from build123d import *

# Parameters (mm, degrees)
BODY_SKETCH_W                                = 46
BODY_SKETCH_H                                = 17
BODY_DEPTH                                   = 105
BODY_ROD_HOLES_SKETCH_R                      = 3
BODY_ROD_HOLES_DEPTH                         = 10
BODY_PISTON_HOLES_SKETCH_R                   = 4.05
BODY_PISTON_HOLES_DEPTH                      = 51
TOP_SWITCH_GROOVES_DEPTH                     = 108.953693777
SHCS_MGT_HOLE_CHAM_SIZE                      = 0.3
SHCS_MGT_HOLE_PAT_COUNT                      = 2
SHCS_MGT_HOLE_PAT_PITCH                      = 40
SHCS_MGT_HOLE_CHAM_OF_SHCS_MGT_HOLE_PAT_SIZE = 0.3
SHCS_MGT_HOLE_BOT_TAP_AT_2_COUNT             = 2
SHCS_MGT_HOLE_BOT_TAP_AT_2_PITCH             = 40
ADJUSTER_NUT_DEPTH                           = 9
ADJUSTER_NUT_THREADS_SKETCH_W                = 1.4
ADJUSTER_NUT_THREADS_SKETCH_H                = 17
TAP_DRILL_FOR_M5X0_8_TAP1_D                  = 4.2
TAP_DRILL_FOR_M5X0_8_TAP1_DEPTH              = 4.5
TAP_DRILL_FOR_M5X0_8_TAP1_CSINK_D            = 5
TAP_DRILL_FOR_M5X0_8_TAP1_CSINK_ANGLE        = 90
TAP_DRILL_FOR_M5X0_8_TAP1_TIP                = 1.2618073
TAP_DRILL_FOR_M5X0_8_TAP2_D                  = 4.2
TAP_DRILL_FOR_M5X0_8_TAP2_DEPTH              = 4.5
TAP_DRILL_FOR_M5X0_8_TAP2_CSINK_D            = 5
TAP_DRILL_FOR_M5X0_8_TAP2_CSINK_ANGLE        = 90
TAP_DRILL_FOR_M5X0_8_TAP2_TIP                = 1.2618073
MOUNT_HOLES_1_D                              = 2.5
MOUNT_HOLES_1_DEPTH                          = 4.5
MOUNT_HOLES_1_CSINK_D                        = 3
MOUNT_HOLES_1_CSINK_ANGLE                    = 90
MOUNT_HOLES_1_TIP                            = 0.751075774
MOUNT_HOLES_2_D                              = 2.5
MOUNT_HOLES_2_DEPTH                          = 4.5
MOUNT_HOLES_2_CSINK_D                        = 3
MOUNT_HOLES_2_CSINK_ANGLE                    = 90
MOUNT_HOLES_2_TIP                            = 0.751075774


with BuildPart() as part:
    # Body_Sketch → Body (new body)
    with BuildSketch(Plane(origin=(0, 0, 0), x_dir=(0, 0, -1), z_dir=(1, 0, 0))):
        with Locations((0, 1.5)):
            Rectangle(BODY_SKETCH_W, BODY_SKETCH_H)
    extrude(amount=BODY_DEPTH)

    # Body Rod Holes_Sketch → Body Rod Holes (cut)
    with BuildSketch(Plane.ZY):
        with Locations((-10, 0)):
            Circle(BODY_ROD_HOLES_SKETCH_R)
        with Locations(Location((10, 0, 0), (0, 0, 180))):
            Circle(BODY_ROD_HOLES_SKETCH_R)
    extrude(amount=-BODY_ROD_HOLES_DEPTH, mode=Mode.SUBTRACT)

    # Body Piston Holes_Sketch → Body Piston Holes (cut)
    with BuildSketch(Plane.ZY.offset(-10)):
        with Locations((10, 0)):
            Circle(BODY_PISTON_HOLES_SKETCH_R)
        with Locations((-10, 0)):
            Circle(BODY_PISTON_HOLES_SKETCH_R)
    extrude(amount=-BODY_PISTON_HOLES_DEPTH, mode=Mode.SUBTRACT)

    # Top Switch Grooves_Sketch → Top Switch Grooves (cut, through all)
    with BuildSketch(Plane.ZY):
        Polygon((13.65, 5.2), (19.95, 5.2), (19.95, 8.8), (19.3, 9.175277675), (19.3, 10), (14.3, 10), (14.3, 9.175277675), (13.65, 8.8), align=None)
        Polygon((-13.65, 8.8), (-13.65, 5.2), (-19.95, 5.2), (-19.95, 8.8), (-19.3, 9.175277675), (-19.3, 10), (-14.3, 10), (-14.3, 9.175277675), align=None)
    extrude(amount=-TOP_SWITCH_GROOVES_DEPTH, mode=Mode.SUBTRACT)

    # SHCS MGT Hole_Sketch → SHCS MGT Hole (revolve, cut)
    with BuildSketch(Plane.XY, mode=Mode.PRIVATE) as shcs_mgt_hole_sk:
        Polygon((20, 10), (16.75, 10), (16.75, 6.7), (18.3, 6.7), (18.3, -7), (20, -7), align=None)
    shcs_mgt_hole = revolve(shcs_mgt_hole_sk.sketch.rotate(Axis((20, -11.506886035, 0), (0, 1, 0)), 270), axis=Axis((20, -11.506886035, 0), (0, 1, 0)), mode=Mode.SUBTRACT)

    # SHCS MGT Hole Cham
    shcs_mgt_hole_cham_edges = [part.edges().sort_by_distance(p)[0] for p in [
        (20, 10, 3.25),
    ]]
    chamfer(shcs_mgt_hole_cham_edges, length=SHCS_MGT_HOLE_CHAM_SIZE)

    # SHCS MGT Hole Pat: SHCS MGT Hole ×2
    with Locations(*[(i * SHCS_MGT_HOLE_PAT_PITCH, 0, 0) for i in range(1, SHCS_MGT_HOLE_PAT_COUNT)]):
        add(shcs_mgt_hole, mode=Mode.SUBTRACT)

    # SHCS MGT Hole Cham of SHCS MGT Hole Pat
    shcs_mgt_hole_cham_of_shcs_mgt_hole_pat_edges = [part.edges().sort_by_distance(p)[0] for p in [
        (60, 10, 3.25),
    ]]
    chamfer(shcs_mgt_hole_cham_of_shcs_mgt_hole_pat_edges, length=SHCS_MGT_HOLE_CHAM_OF_SHCS_MGT_HOLE_PAT_SIZE)

    # SHCS MGT Hole Bot Tap Profile → SHCS MGT Hole Bot Tap (revolve, cut)
    with BuildSketch(Plane(origin=(20, -7, 0), x_dir=(0, 0, -1), z_dir=(1, 0, 0))):
        Polygon((0, 0), (0, 9.021463052), (1.7, 8), (1.7, 7), (2, 7), (2, 0.3), (2.3, 0), align=None)
    shcs_mgt_hole_bot_tap = revolve(axis=Axis((20, -13.35, 0), (0, 1, 0)), mode=Mode.SUBTRACT)

    # SHCS MGT Hole Bot Tap at 2: SHCS MGT Hole Bot Tap ×2
    with Locations(*[(i * SHCS_MGT_HOLE_BOT_TAP_AT_2_PITCH, 0, 0) for i in range(1, SHCS_MGT_HOLE_BOT_TAP_AT_2_COUNT)]):
        add(shcs_mgt_hole_bot_tap, mode=Mode.SUBTRACT)

    # Adjuster Nut_Sketch → Adjuster Nut (add)
    with BuildSketch(Plane.ZY):
        Polygon((-2.020725942, 8.5), (2.020725942, 8.5), (4.041451884, 5), (2.020725942, 1.5), (-2.020725942, 1.5), (-4.041451884, 5), align=None)
    extrude(amount=ADJUSTER_NUT_DEPTH)

    # Adjuster Nut Threads_Sketch → Adjuster Nut Threads (revolve, cut)
    with BuildSketch(Plane.XY, mode=Mode.PRIVATE) as adjuster_nut_threads_sk:
        with Locations((-3.9, 15.5)):
            Rectangle(ADJUSTER_NUT_THREADS_SKETCH_W, ADJUSTER_NUT_THREADS_SKETCH_H)
    revolve(adjuster_nut_threads_sk.sketch.rotate(Axis((-6.476, 5, 0), (1, 0, 0)), 270), axis=Axis((-6.476, 5, 0), (1, 0, 0)), mode=Mode.SUBTRACT)

    # Tap Drill for M5x0.8 Tap1
    with Locations(Plane.XY.offset(23)):
        with Locations((30, 0), (97, 0)):
            CounterSinkHole(TAP_DRILL_FOR_M5X0_8_TAP1_D / 2, TAP_DRILL_FOR_M5X0_8_TAP1_CSINK_D / 2, depth=TAP_DRILL_FOR_M5X0_8_TAP1_DEPTH, counter_sink_angle=TAP_DRILL_FOR_M5X0_8_TAP1_CSINK_ANGLE)
            with Locations((0, 0, -(TAP_DRILL_FOR_M5X0_8_TAP1_DEPTH + TAP_DRILL_FOR_M5X0_8_TAP1_TIP / 2))):  # 118° drill point
                Cone(0, TAP_DRILL_FOR_M5X0_8_TAP1_D / 2, TAP_DRILL_FOR_M5X0_8_TAP1_TIP, mode=Mode.SUBTRACT)

    # Tap Drill for M5x0.8 Tap2
    with Locations(Plane(origin=(0, 0, -23), x_dir=(-1, 0, 0), z_dir=(0, 0, -1))):
        with Locations((-97, 0), (-30, 0)):
            CounterSinkHole(TAP_DRILL_FOR_M5X0_8_TAP2_D / 2, TAP_DRILL_FOR_M5X0_8_TAP2_CSINK_D / 2, depth=TAP_DRILL_FOR_M5X0_8_TAP2_DEPTH, counter_sink_angle=TAP_DRILL_FOR_M5X0_8_TAP2_CSINK_ANGLE)
            with Locations((0, 0, -(TAP_DRILL_FOR_M5X0_8_TAP2_DEPTH + TAP_DRILL_FOR_M5X0_8_TAP2_TIP / 2))):  # 118° drill point
                Cone(0, TAP_DRILL_FOR_M5X0_8_TAP2_D / 2, TAP_DRILL_FOR_M5X0_8_TAP2_TIP, mode=Mode.SUBTRACT)

    # Mount_Holes_1
    with Locations(Plane.XY.offset(23)):
        with Locations((20, 1.5), (60, 1.5)):
            CounterSinkHole(MOUNT_HOLES_1_D / 2, MOUNT_HOLES_1_CSINK_D / 2, depth=MOUNT_HOLES_1_DEPTH, counter_sink_angle=MOUNT_HOLES_1_CSINK_ANGLE)
            with Locations((0, 0, -(MOUNT_HOLES_1_DEPTH + MOUNT_HOLES_1_TIP / 2))):  # 118° drill point
                Cone(0, MOUNT_HOLES_1_D / 2, MOUNT_HOLES_1_TIP, mode=Mode.SUBTRACT)

    # Mount_Holes_2
    with Locations(Plane(origin=(0, 0, -23), x_dir=(-1, 0, 0), z_dir=(0, 0, -1))):
        with Locations((-60, 1.5), (-20, 1.5)):
            CounterSinkHole(MOUNT_HOLES_2_D / 2, MOUNT_HOLES_2_CSINK_D / 2, depth=MOUNT_HOLES_2_DEPTH, counter_sink_angle=MOUNT_HOLES_2_CSINK_ANGLE)
            with Locations((0, 0, -(MOUNT_HOLES_2_DEPTH + MOUNT_HOLES_2_TIP / 2))):  # 118° drill point
                Cone(0, MOUNT_HOLES_2_D / 2, MOUNT_HOLES_2_TIP, mode=Mode.SUBTRACT)


solid = part.part
Verification items for the finished model (mm, model axes). A direction names the side the tool comes from. Coordinates: 2 decimals unless noted, no trailing zeros. Order: outer loops, then holes, each group sorted by start corner. A loop starts at its lowest first (then second) coordinate and runs counter-clockwise, first axis right, second up. Notation, with made-up numbers: M 14,58.25 L 51,58.25 A15 cw 51,64.25 Z; hole C -15,53.25 d4. An arc over 180 degrees is marked long. One line per item, written item: value. Start each with the question number.
Item 1: Depth check by flat-ended pin: P1, Ø2, axis at x = -8, z = -0.5, coming from the +Y side; P2, Ø3, axis at x = 59.5, z = 1, coming from the +Y side; P3, Ø4, axis at y = 1, z = 4.5, coming from the -X side; P4, Ø2, axis at x = 60, z = 0, coming from the +Y side. Enter the tip coordinate at first touch or a pass-through.
Item 2: Mould release check, pull along Z, two halves, no side actions. Record for faces 5 (the conical face through (30.364, 0.016, -17.457)), 6 (the flat face through (52, 5.2, -17)), 7 (the flat face through (-7, 8.5, 0)): pulls with the +Z half, pulls with the -Z half, needs draft (parallel to the pull), parting line crosses it, or undercut.
Item 3: Sectioned sample at B-B on z = 10. Record the cut outline in (x, y).
Item 4: Sectioned sample at D-D on z = 0. Give the number of separate pieces and of enclosed holes in the cut face, then the cut area to 3 significant figures.
Item 5: Sectioned sample at A-A on x = 44.5. Record the cut outline in (y, z).
Item 6: Thickness scan on probe 1 along X at (y, z) = (5.75, 0); probe 2 along X at (y, z) = (-4.75, 0); probe 3 along X at (y, z) = (-1.25, 7). Record the ranges inside material, lowest first.
Item 7: Access from +Z, -Z, +X, -X, +Y, -Y to the whole of each face (thin tool, end or side, straight path). Record for faces 1 (the flat face through (-4.6, 7, 2)), 2 (the flat face through (52, 7, 13.65)), 3 (the cylindrical face through (56.778, 8.179, 0.423)), 4 (the flat face through (-6.769, 3.274, 3.045)).
Item 8: Sectioned sample at C-C on x = 71. Record the cut outline in (y, z), then the cut area to 3 significant figures.
Calculated:
1. P1: y = 8.5
1. P2: y = 6.7
1. P3: x = 0
1. P4: through
2. face 5: pulls with the -Z half
2. face 6: undercut
2. face 7: needs draft
3. outline: M 0,-7 L 105,-7 L 105,10 L 0,10 L 0,3 L 10,3 L 10,4.05 L 61,4.05 L 61,-4.05 L 10,-4.05 L 10,-3 L 0,-3 Z
4. separate pieces: 3
4. enclosed holes: 0
4. area: 1,700 mm^2
5. outline: M -7,-23 L 10,-23 L 10,-19.3 L 9.18,-19.3 L 8.8,-19.95 L 5.2,-19.95 L 5.2,-13.65 L 8.8,-13.65 L 9.18,-14.3 L 10,-14.3 L 10,14.3 L 9.18,14.3 L 8.8,13.65 L 5.2,13.65 L 5.2,19.95 L 8.8,19.95 L 9.18,19.3 L 10,19.3 L 10,23 L -7,23 Z; hole C 0,-10 d8.1; hole C 0,10 d8.1
6. probe 1: -9 to 18.3, 21.7 to 58.3, 61.7 to 105
6. probe 2: 0 to 18, 22 to 58, 62 to 105
6. probe 3: 0 to 10, 61 to 105
7. face 1: none
7. face 2: +X, -X
7. face 3: +Y
7. face 4: +Z, -X, -Y
8. outline: M -7,-23 L 10,-23 L 10,-19.3 L 9.18,-19.3 L 8.8,-19.95 L 5.2,-19.95 L 5.2,-13.65 L 8.8,-13.65 L 9.18,-14.3 L 10,-14.3 L 10,14.3 L 9.18,14.3 L 8.8,13.65 L 5.2,13.65 L 5.2,19.95 L 8.8,19.95 L 9.18,19.3 L 10,19.3 L 10,23 L -7,23 Z
8. area: 724 mm^2
